Read the model definition and answer for the solid it produces. Units are mm, in the model's axes. A direction names the side the tool comes from. Coordinates: 2 decimals unless noted, no trailing zeros. Loops run counter-clockwise (first coordinate to the right, second up) from the corner with the lowest first, then second, coordinate; pieces in that order, holes last.
Q1. Section C-C (y = 3.5) is taken. Give the vertices of the cut face in (x, z).
Q2. The mould has two halves that part along Z. Classify faces 3 (the face through (2.43, 6.26, -2.23)), 4 (the face through (-3, 12.7, 2)): pulls with the +Z half, pulls with the -Z half, needs draft (parallel to the pull), parting line crosses it, or undercut.
Q3. Section B-B (z = 0) is taken. Give the vertices of the cut face in (x, y).
Q4. Flat-ended cylindrical pins translate along their axes: P1, Ø2, axis at y = 11, z = -2, coming from the +X side; P2, Ø3, axis at x = -3.5, y = 9, coming from the +Z side. Find the tip coordinate at first contact, or state that the pin passes through.
Q5. Section A-A (x = 0) is taken. Give the vertices of the cut face in (y, z).
Q6. Straight lines are drawn through the part: line 1 (Z direction, x = 0, y = 8.25); line 2 (Z direction, x = 0, y = 3.25); line 3 (Y direction, x = -3.25, z = -3). For each, find the intervals that lie inside material, in ascending order.
Q7. Section D-D (z = 1.5) is taken. Give the vertices of the cut face in (x, y).
Q8. Which of the six approach directions +Z, -Z, +X, -X, +Y, -Y give full straight-line access (tool end or side, diameter ignored) to faces 1 (the face through (3, 0, 2)), 2 (the face through (-4.247, 6.261, -0.943))?
from build123d import *

# Parameters (mm, degrees)
SKETCH1_R            = 4.35
BODY_DEPTH           = 12.7
TEETH_START          = -7.7
TEETH_DEPTH          = 7.7
CIRPATTERN1_COUNT    = 15
M6_CLEARANCE_HOLE1_D = 6.6


with BuildPart() as part:
    # Sketch1 → Body (new body)
    with BuildSketch(Plane(origin=(0, 0, 0), x_dir=(1, 0, 0), z_dir=(0, 1, 0))):
        with Locations(Location((0, 0, 0), (0, 0, 270))):
            Circle(SKETCH1_R)
    extrude(amount=BODY_DEPTH)

    # Sketch2 → Teeth (add)
    with BuildSketch(Plane(origin=(0, 12.7, 0), x_dir=(1, 0, 0), z_dir=(0, 1, 0)).offset(TEETH_START)):
        with BuildLine():
            Line((-0.2, 4.345399867), (-0.2, 4.445399867))
            Line((-0.2, 4.445399867), (0.2, 4.445399867))
            Line((0.2, 4.445399867), (0.2, 4.345399867))
            ThreePointArc((0.2, 4.345399867), (0, 4.35), (-0.2, 4.345399867))
        make_face()
    teeth = extrude(amount=TEETH_DEPTH)

    # CirPattern1: Teeth ×15 about axis
    cirpattern1_axis = Axis((0, 0, 0), (0, 1, 0))
    for i in range(1, CIRPATTERN1_COUNT):
        add(teeth.rotate(cirpattern1_axis, i * 360 / CIRPATTERN1_COUNT))

    # M6 Clearance Hole1 (through all)
    with Locations(Plane(origin=(0, 12.7, 0), x_dir=(1, 0, 0), z_dir=(0, 1, 0))):
        with Locations((0, 0)):
            Hole(M6_CLEARANCE_HOLE1_D / 2)


solid = part.part
Numbers:
1. outline: circle Ø8.7 at (0, 0); hole circle Ø6.6 at (0, 0)
2. face 3: undercut
2. face 4: needs draft
3. outline: (-4.35, 0) - (-3.3, 0) - (-3.3, 12.7) - (-4.35, 12.7) - close; (3.3, 0) - (4.35, 0) - (4.35, 12.7) - (3.3, 12.7) - close
4. P1: stops at x = 4.29
4. P2: stops at z = 3.86
5. outline: (0, -4.35) - (5, -4.35) - (5, -4.45) - (12.7, -4.45) - (12.7, -3.3) - (0, -3.3) - close; (0, 3.3) - (12.7, 3.3) - (12.7, 4.35) - (0, 4.35) - close
6. line 1: z = -4.45 to -3.3, 3.3 to 4.35
6. line 2: z = -4.35 to -3.3, 3.3 to 4.35
6. line 3: y = 5 to 12.7
7. outline: (-4.08, 0) - (-2.94, 0) - (-2.94, 12.7) - (-4.08, 12.7) - close; (2.94, 0) - (4.08, 0) - (4.08, 12.7) - (2.94, 12.7) - close
8. face 1: +Z, -Z, +X, -X, -Y
8. face 2: -Y
